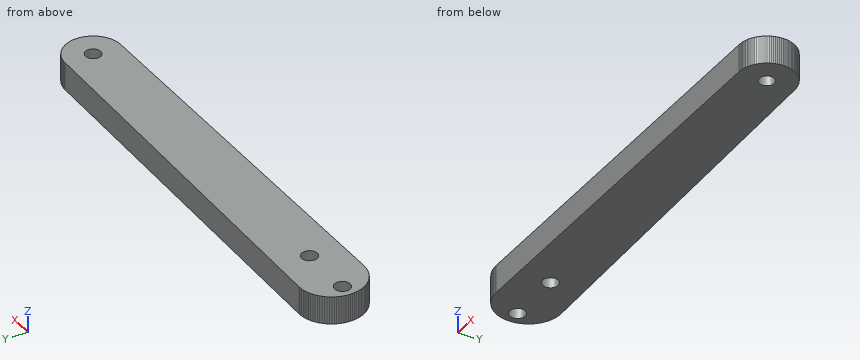
```python
from build123d import *

# Parameters (mm, degrees)
PLATE_DEPTH       = 6
SKETCH2_R         = 1.7
HUB_SCREWS_DEPTH  = 6
SKETCH3_R         = 1.65
KNOB_THREAD_DEPTH = 6


with BuildPart() as part:
    # Sketch1 → Plate (new body)
    with BuildSketch(Plane.XY):
        Polygon((-2, 7), (-2.457821905, 6.985012463), (-2.913683346, 6.94011403), (-3.365632254, 6.865496963), (-3.811733316, 6.761480784), (-4.250076257, 6.628510906), (-4.678784027, 6.467156728), (-5.096020832, 6.278109191), (-5.5, 6.062177826), (-5.888991631, 5.820287286), (-6.261330003, 5.553473382), (-6.615420706, 5.262878652), (-6.949747468, 4.949747468), (-7.262878652, 4.615420706), (-7.553473382, 4.261330003), (-7.820287286, 3.888991631), (-8.062177826, 3.5), (-8.278109191, 3.096020832), (-8.467156728, 2.678784027), (-8.628510906, 2.250076257), (-8.761480784, 1.811733316), (-8.865496963, 1.365632254), (-8.94011403, 0.913683346), (-8.985012463, 0.457821905), (-9, 0), (-8.985012463, -0.457821905), (-8.94011403, -0.913683346), (-8.865496963, -1.365632254), (-8.761480784, -1.811733316), (-8.628510906, -2.250076257), (-8.467156728, -2.678784027), (-8.278109191, -3.096020832), (-8.062177826, -3.5), (-7.820287286, -3.888991631), (-7.553473382, -4.261330003), (-7.262878652, -4.615420706), (-6.949747468, -4.949747468), (-6.615420706, -5.262878652), (-6.261330003, -5.553473382), (-5.888991631, -5.820287286), (-5.5, -6.062177826), (-5.096020832, -6.278109191), (-4.678784027, -6.467156728), (-4.250076257, -6.628510906), (-3.811733316, -6.761480784), (-3.365632254, -6.865496963), (-2.913683346, -6.94011403), (-2.457821905, -6.985012463), (-2, -7), (85, -6), (85.392418775, -5.987153539), (85.783157153, -5.948669168), (86.170541932, -5.884711682), (86.552914271, -5.795554958), (86.928636792, -5.681580777), (87.296100594, -5.543277195), (87.653732141, -5.381236449), (88, -5.196152423), (88.333421398, -4.988817674), (88.652568574, -4.760120042), (88.956074891, -4.511038845), (89.242640687, -4.242640687), (89.511038845, -3.956074891), (89.760120042, -3.652568574), (89.988817674, -3.333421398), (90.196152423, -3), (90.381236449, -2.653732141), (90.543277195, -2.296100594), (90.681580777, -1.928636792), (90.795554958, -1.552914271), (90.884711682, -1.170541932), (90.948669168, -0.783157153), (90.987153539, -0.392418775), (91, 0), (90.987153539, 0.392418775), (90.948669168, 0.783157153), (90.884711682, 1.170541932), (90.795554958, 1.552914271), (90.681580777, 1.928636792), (90.543277195, 2.296100594), (90.381236449, 2.653732141), (90.196152423, 3), (89.988817674, 3.333421398), (89.760120042, 3.652568574), (89.511038845, 3.956074891), (89.242640687, 4.242640687), (88.956074891, 4.511038845), (88.652568574, 4.760120042), (88.333421398, 4.988817674), (88, 5.196152423), (87.653732141, 5.381236449), (87.296100594, 5.543277195), (86.928636792, 5.681580777), (86.552914271, 5.795554958), (86.170541932, 5.884711682), (85.783157153, 5.948669168), (85.392418775, 5.987153539), (85, 6), align=None)
    extrude(amount=PLATE_DEPTH)

    # Sketch2 → Hub_screws (cut)
    with BuildSketch(Plane.XY):
        with Locations((-6, 0)):
            Circle(SKETCH2_R)
        with Locations((6, 0)):
            Circle(SKETCH2_R)
    extrude(amount=HUB_SCREWS_DEPTH, mode=Mode.SUBTRACT)

    # Sketch3 → Knob_thread (cut)
    with BuildSketch(Plane.XY):
        with Locations((85, 0)):
            Circle(SKETCH3_R)
    extrude(amount=KNOB_THREAD_DEPTH, mode=Mode.SUBTRACT)


solid = part.part
```
Check sheet for the modelled part. Datum: model origin and axes. Units: mm. Round coordinates to 2 decimals unless told otherwise and drop trailing zeros. Loops run counter-clockwise (first coordinate to the right, second up) from the corner with the lowest first, then second, coordinate; pieces in that order, holes last. Notation, with made-up numbers: (-10, -40) - (43, -40) arc R27 cw to (43, -10) - close; hole circle Ø8 at (69.5, -16). An arc over 180 degrees is marked (long way). Answer as a JSON object with one key per item and string values. Group by question number.
Q1. Sectioned sample at B-B, the plane z = 2.75. Count the separate pieces of the cut face and the enclosed holes in it, plus the area to 3 significant figures.
Q2. Scan lines: line 1 along X through (y, z) = (-0.25, 3.35); line 2 along X through (y, z) = (-0.75, 3.1); line 3 along Y through (x, z) = (46, 5.6). Record each from-to range of solid material in increasing order. Write a range as [from, to].
Q3. Gauge pin test, flat ends, axial feed: P1, Ø4.5, axis at x = 85, y = 0, coming from the -Z side; P2, Ø1, axis at x = 51.5, z = 2.5, coming from the +Y side; P3, Ø1.5, axis at x = 80, z = 1, coming from the +Y side. Record the tip position at first contact, or that the pin passes through.
Q4. Sectioned sample at A-A, the plane x = 6. Enter the section's corners in (y, z), plus the area to 3 significant figures.
Q5. Sectioned sample at C-C, the plane x = 72.5. Enter the section's corners in (y, z), plus the area to 3 significant figures.
Q6. Sectioned sample at D-D, the plane x = 58. Enter the section's corners in (y, z).
Solution:
{
 "1": {"separate pieces": "1", "enclosed holes": "3", "area": "1,240 mm²"},
 "2": {"line 1": "x = [-8.99, -7.68], [-4.32, 4.32], [7.68, 83.37], [86.63, 90.99]", "line 2": "x = [-8.96, -7.53], [-4.47, 4.47], [7.53, 83.53], [86.47, 90.95]", "line 3": "y = [-6.45, 6.45]"},
 "3": {"P1": "stops at z = 0", "P2": "stops at y = 6.39", "P3": "stops at y = 6.07"},
 "4": {"outline": "(-6.91, 0) - (-1.7, 0) - (-1.7, 6) - (-6.91, 6) - close; (1.7, 0) - (6.91, 0) - (6.91, 6) - (1.7, 6) - close", "area": "62.5 mm²"},
 "5": {"outline": "(-6.14, 0) - (6.14, 0) - (6.14, 6) - (-6.14, 6) - close", "area": "73.7 mm²"},
 "6": {"outline": "(-6.31, 0) - (6.31, 0) - (6.31, 6) - (-6.31, 6) - close"}
}
